Design review of the part built by this model. Coordinates are the model's own, in mm. A direction names the side the tool comes from. Coordinates: 2 decimals unless noted, no trailing zeros. Loops run counter-clockwise (first coordinate to the right, second up) from the corner with the lowest first, then second, coordinate; pieces in that order, holes last. Notation, with made-up numbers: (-37.5, 88.25) - (6.5, 88.25) arc R10 ccw to (6.5, 106.25) - close; hole circle Ø2 at (31, 87.5). An arc over 180 degrees is marked (long way). One line per question, with ' | ' between items.
from build123d import *

# Parameters (mm, degrees)
F3_R = 5


with BuildPart() as f2:
    # F2: sweep along a path in F0
    with BuildLine(Plane.XY) as f2_path:
        Line((0, -50), (-20, -30))
        Line((-20, -30), (-20, 30))
        Line((-20, 30), (0, 50))
    # F1 (on Front) → F2 (sweep)
    with BuildSketch(Plane.XZ):
        Polygon((-20, 0), (-10, 0), (-10, 2), (-16.7639320225, 2), (-3.7639320225, 28), (5, 28), (5, 30), (-5, 30), align=None)
    sweep(path=f2_path.line, transition=Transition.RIGHT)

    # F3
    f3_edges = [f2.edges().sort_by_distance(p)[0] for p in [
        (-5, 0, 30),
        (2.803301, 31.590097, 30),
        (2.803301, -31.590097, 30),
        (-12.5, -26.893398, 15),
        (-12.5, 26.893398, 15),
    ]]
    fillet(f3_edges, radius=F3_R)


solid = f2.part
Q1. To check wall thickness, follow line 1 along Y through (x, z) = (1.5, 21); line 2 along Y through (x, z) = (-4, 16); line 3 along Z through (x, y) = (0.5, -21). State the ranges of each line that lie inside material, in increasing order.
Returned:
line 1: y = -36.65 to -33.49, 33.49 to 36.65 | line 2: y = -34.69 to -31.52, 31.52 to 34.69 | line 3: z = 28 to 30
Q2. Tool access review of faces 4 (the flat face through (-1.584, -34.274, 0.986)), 5 (the flat face through (-13, -2, 0)), 6 (the flat face through (-10.355, 0.401, 14.818)), 7 (the flat face through (11.428, 26.072, 28.986)), 8 (the cylindrical face through (-12.92, -27.09, 13.47)): name each direction out of +Z, -Z, +X, -X, +Y, -Y from which nothing blocks a thin tool from reaching the whole face with its end or side.
Returned:
face 4: -Z, +X | face 5: -Z, +X, -X, +Y, -Y | face 6: +X | face 7: +Z, -Z, +X | face 8: +Z, -X, -Y
Q3. Draft analysis for pull direction Z (two halves, no side actions). For faces 1 (the flat face through (-2.84, -33.52, 14.82)), 2 (the flat face through (-10, 0, 1)), 3 (the cylindrical face through (3.708, 31.796, 29.273)), state which applies: +Z half, -Z half, draft (parallel to the pull), parting line (faces both ways), or undercut.
Returned:
face 1: undercut | face 2: draft | face 3: +Z half
Q4. Take a section at A-A (x = 15.5). Give the boundary of the cut face in (y, z), plus the area to 3 significant figures.
Returned:
outline: (-34.5, 28) - (-30.14, 28) - (-30.14, 30) - (-34.5, 30) - close; (30.14, 28) - (34.5, 28) - (34.5, 30) - (30.14, 30) - close | area: 17.4 mm²
Q5. Take a section at B-B (y = -6.5). Give the boundary of the cut face in (x, z), plus the area to 3 significant figures.
Returned:
outline: (-20, 0) - (-10, 0) - (-10, 2) - (-16.76, 2) - (-3.76, 28) - (5, 28) - (5, 30) - (-1.91, 30) arc R5 ccw to (-6.38, 27.24) - close | area: 96.5 mm²
Q6. For pin 1 (1.5 mm diameter, centred on x = 4.5, y = -14.5, fed in from -Z); pin 2 (5 mm diameter, centred on y = 28.5, z = 5.5, fed in from +X); pin 3 (1.5 mm diameter, centred on y = 0.5, z = 21.5, fed in from +X); pin 4 (7 mm diameter, centred on x = -5.5, y = -13, fed in from +Z), all flat-tipped, find the tip position at first contact; note any pin that passes through.
Returned:
pin 1: stops at z = 28 | pin 2: stops at x = -11.39 | pin 3: stops at x = -6.64 | pin 4: stops at z = 30
